Here's how the part is built. I have some questions about the finished solid (model axes, mm). Face numbers are marked on the shaded views. A direction names the side the tool comes from. Round coordinates to 2 decimals unless told otherwise and drop trailing zeros. Write each loop counter-clockwise with the first axis right and the second up, starting at its lowest first coordinate (ties: lowest second). Pieces come first, ordered by that corner, then holes. Notation, with made-up numbers: (-38.5, 25.5) - (-17.5, 25.5) arc R15 ccw to (-17.5, 45.5) - close; hole circle Ø2 at (19.5, 28.25). An arc over 180 degrees is marked (long way). Use one line per item in the form item = value. Start each with the question number.
1. I want a section at C-C, the plane y = 1. List the corners of the cut face in (x, z) for me, plus the area to 3 significant figures.
2. If I drill on line 1 along X through (y, z) = (5.9, 0); line 2 along X through (y, z) = (1.1, 0); line 3 along Y through (x, z) = (2.5, 5.25), over which ranges is the centre line in solid material (lowest first)?
3. Which directions (+Z, -Z, +X, -X, +Y, -Y) give clear straight access to the entire face, cutting with the end or side of a thin tool? Please do the marked faces 4 and 5.
4. We'd pull the mould along X, two halves only. Please class the marked faces 1, 2 and 3: +X half, -X half, draft (parallel to the pull), parting line (faces both ways), or undercut.
5. Will these pins go through, and if not, where does the flat tip stop? pin 1 (2 mm diameter, centred on x = 16, y = 2, fed in from -Z); pin 2 (4 mm diameter, centred on x = -3.5, y = 4, fed in from -Z).
6. I want a section at B-B, the plane z = 0. List the corners of the cut face in (x, y) for me, plus the area to 3 significant figures.
7. I want a section at D-D, the plane x = -5.5. List the corners of the cut face in (y, z) for me, plus the area to 3 significant figures.
8. I want a section at A-A, the plane x = 0.9. List the corners of the cut face in (y, z) for me, plus the area to 3 significant figures.
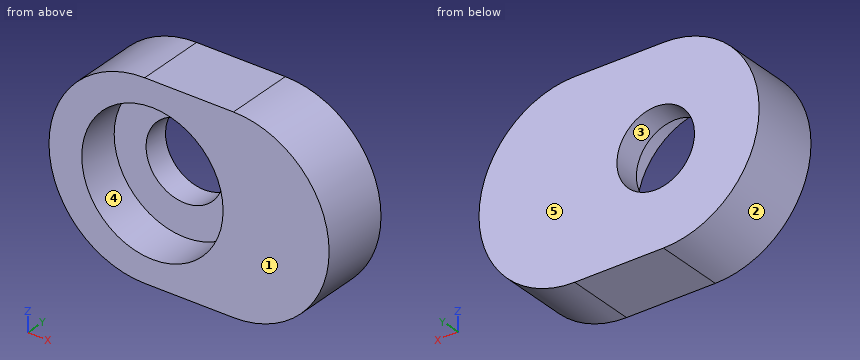
```python
from build123d import *

# Parameters (mm, degrees)
SKETCH1_R           = 8.2
BOSS_EXTRUDE1_DEPTH = 8
BOSS_EXTRUDE2_START = -3
SKETCH2_R           = 8.2
SKETCH2_R_2         = 4.5
BOSS_EXTRUDE2_DEPTH = 3


with BuildPart() as part:
    # Sketch1 → Boss-Extrude1 (new body)
    with BuildSketch(Plane(origin=(0, 0, 0), x_dir=(1, 0, 0), z_dir=(0, 1, 0))):
        with BuildLine():
            Line((0, 11.1), (10.3, 11.1))
            ThreePointArc((10.3, 11.1), (21.4, 0), (10.3, -11.1))
            Line((10.3, -11.1), (0, -11.1))
            ThreePointArc((0, -11.1), (-11.1, 0), (0, 11.1))
        make_face()
        with Locations(Location((0.9, 0, 0), (0, 0, 270))):
            Circle(SKETCH1_R, mode=Mode.SUBTRACT)
    extrude(amount=BOSS_EXTRUDE1_DEPTH)

    # Sketch2 → Boss-Extrude2 (add)
    with BuildSketch(Plane(origin=(0, 8, 0), x_dir=(1, 0, 0), z_dir=(0, 1, 0)).offset(BOSS_EXTRUDE2_START)):
        with Locations(Location((0.9, 0, 0), (0, 0, 270))):
            Circle(SKETCH2_R)
        with Locations(Location((0.9, 0, 0), (0, 0, 270))):
            Circle(SKETCH2_R_2, mode=Mode.SUBTRACT)
    extrude(amount=BOSS_EXTRUDE2_DEPTH)


solid = part.part
```
Model answer:
q1.outline = (0, -11.1) - (10.3, -11.1) arc R11.1 ccw to (10.3, 11.1) - (0, 11.1) arc R11.1 ccw to start; hole circle Ø16.4 at (0.9, 0)
q1.area = 404 mm2
q2.line_1 = -11.1 to -3.6, 5.4 to 21.4
q2.line_2 = -11.1 to -7.3, 9.1 to 21.4
q2.line_3 = 5 to 8
q3.face_4 = -Y
q3.face_5 = +Z, -Z, +X, -X, +Y
q4.face_1 = draft
q4.face_2 = -X half
q4.face_3 = undercut
q5.pin_1 = -10.06
q5.pin_2 = -11
q6.outline = (-11.1, 0) - (-7.3, 0) - (-7.3, 5) - (-3.6, 5) - (-3.6, 8) - (-11.1, 8) - close; (5.4, 5) - (9.1, 5) - (9.1, 0) - (21.4, 0) - (21.4, 8) - (5.4, 8) - close
q6.area = 151 mm2
q7.outline = (0, -9.64) - (8, -9.64) - (8, 9.64) - (0, 9.64) - (0, 5.13) - (5, 5.13) - (5, -5.13) - (0, -5.13) - close
q7.area = 103 mm2
q8.outline = (0, -11.1) - (8, -11.1) - (8, -4.5) - (5, -4.5) - (5, -8.2) - (0, -8.2) - close; (0, 8.2) - (5, 8.2) - (5, 4.5) - (8, 4.5) - (8, 11.1) - (0, 11.1) - close
q8.area = 68.6 mm2
